Input: dimensioned drawing with shaded views. Units: mm. Origin: part minimum x, y, z. Round coordinates to 2 decimals unless told otherwise and drop trailing zeros. Write each loop counter-clockwise with the first axis right and the second up, starting at its lowest first coordinate (ties: lowest second). Pieces come first, ordered by that corner, then holes. Notation, with made-up numbers: M 78.25,16.25 L 82.25,16.25 A23 ccw 82.25,24.25 Z; hole C 49,25 d3. An arc over 180 degrees is marked long. Answer as CSV lines item,"result". Start each with the question number.
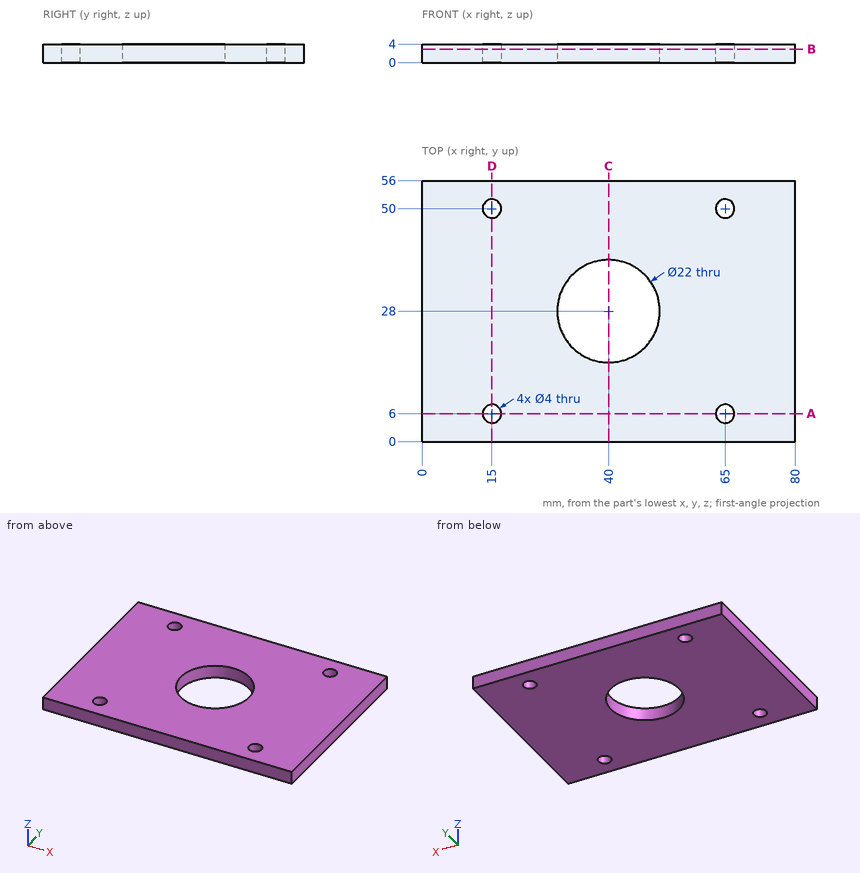
Item 1: Cut plane A-A, the plane y = 6. Return loops of the section in (x, z), plus the area to 3 significant figures.
Item 2: Cut plane C-C, the plane x = 40. Return loops of the section in (y, z).
Item 3: Line query: line 1 (Y direction, x = 65, z = 3.2); line 2 (Y direction, x = 40, z = 0.95); line 3 (X direction, y = 50.5, z = 0.65). Output: solid intervals per line, ascending. Write a range as [from, to].
Item 4: Cut plane D-D, the plane x = 15. Return loops of the section in (y, z), plus the area to 3 significant figures.
Item 5: Cut plane B-B, the plane z = 2.9. Return loops of the section in (x, y), plus the area to 3 significant figures.
Results list:
1,outline,"M 0,0 L 13,0 L 13,4 L 0,4 Z; M 17,0 L 63,0 L 63,4 L 17,4 Z; M 67,0 L 80,0 L 80,4 L 67,4 Z"
1,area,"288 mm²"
2,outline,"M 0,0 L 17,0 L 17,4 L 0,4 Z; M 39,0 L 56,0 L 56,4 L 39,4 Z"
3,line 1,"[0, 4], [8, 48], [52, 56]"
3,line 2,"[0, 17], [39, 56]"
3,line 3,"[0, 13.06], [16.94, 63.06], [66.94, 80]"
4,outline,"M 0,0 L 4,0 L 4,4 L 0,4 Z; M 8,0 L 48,0 L 48,4 L 8,4 Z; M 52,0 L 56,0 L 56,4 L 52,4 Z"
4,area,"192 mm²"
5,outline,"M 0,0 L 80,0 L 80,56 L 0,56 Z; hole C 15,6 d4; hole C 15,50 d4; hole C 40,28 d22; hole C 65,6 d4; hole C 65,50 d4"
5,area,"4,050 mm²"
